Geometry: final body of the model. Coordinates: model frame, mm. Give positions to 0.01 mm unless a question says otherwise; leave off trailing zeros. Order: outer loops, then holes, each group sorted by start corner. A loop starts at its lowest first (then second) coordinate and runs counter-clockwise, first axis right, second up. Notation, with made-up numbers: (16.25, 20) -> (43.25, 20) arc R21 cw to (43.25, 53) -> close; hole circle Ø2 at (83.25, 57). An arc over 180 degrees is marked (long way). One line per question, with ' | ' between items.
from build123d import *

# Parameters (mm, degrees)
SKETCH1_W           = 1.5875
SKETCH1_H           = 1.7272
SKETCH1_R           = 1.0541
SKETCH1_H_2         = 1.778
BOSS_EXTRUDE1_DEPTH = 1.5875


with BuildPart() as part:
    # Sketch1 → Boss-Extrude1 (new body)
    with BuildSketch(Plane.XY):
        with BuildLine():
            Line((-20.6375, 22.848075056), (-20.6375, 0))
            Line((-20.6375, 0), (20.6375, 0))
            Line((20.6375, 0), (20.6375, 38.1))
            Line((20.6375, 38.1), (-20.6375, 38.1))
            Line((-20.6375, 38.1), (-20.6375, 33.337040193))
            ThreePointArc((-20.6375, 33.337040193), (-18.972227818, 30.628064614), (-19.079863508, 27.45))
            Line((-19.079863508, 27.45), (-20.6375, 22.848075056))
        make_face()
        with Locations((-17.68475, 2.977543878)):
            Rectangle(SKETCH1_W, SKETCH1_H, mode=Mode.SUBTRACT)
        with Locations((-18.4658, 14.5415)):
            Circle(SKETCH1_R, mode=Mode.SUBTRACT)
        with Locations((-17.68475, 18.002943878)):
            Rectangle(SKETCH1_W, SKETCH1_H_2, mode=Mode.SUBTRACT)
        with Locations((14.50975, 2.977543878)):
            Rectangle(SKETCH1_W, SKETCH1_H, mode=Mode.SUBTRACT)
        with Locations((14.50975, 18.002943878)):
            Rectangle(SKETCH1_W, SKETCH1_H_2, mode=Mode.SUBTRACT)
        with Locations((18.4658, 14.5415)):
            Circle(SKETCH1_R, mode=Mode.SUBTRACT)
        with BuildLine():
            Line((-8.4, 17), (-8.4, 23.35))
            Line((-8.4, 23.35), (-10.7, 23.35))
            ThreePointArc((-10.7, 23.35), (-12.75, 25.4), (-10.7, 27.45))
            Line((-10.7, 27.45), (-8.4, 27.45))
            Line((-8.4, 27.45), (-8.4, 33.8))
            Line((-8.4, 33.8), (8.4, 33.8))
            Line((8.4, 33.8), (8.4, 27.45))
            Line((8.4, 27.45), (10.7, 27.45))
            ThreePointArc((10.7, 27.45), (12.75, 25.4), (10.7, 23.35))
            Line((10.7, 23.35), (8.4, 23.35))
            Line((8.4, 23.35), (8.4, 17))
            Line((8.4, 17), (-8.4, 17))
        make_face(mode=Mode.SUBTRACT)
        with Locations((-18.4658, 36.2585)):
            Circle(SKETCH1_R, mode=Mode.SUBTRACT)
        with Locations((18.4658, 36.2585)):
            Circle(SKETCH1_R, mode=Mode.SUBTRACT)
    extrude(amount=BOSS_EXTRUDE1_DEPTH)


solid = part.part
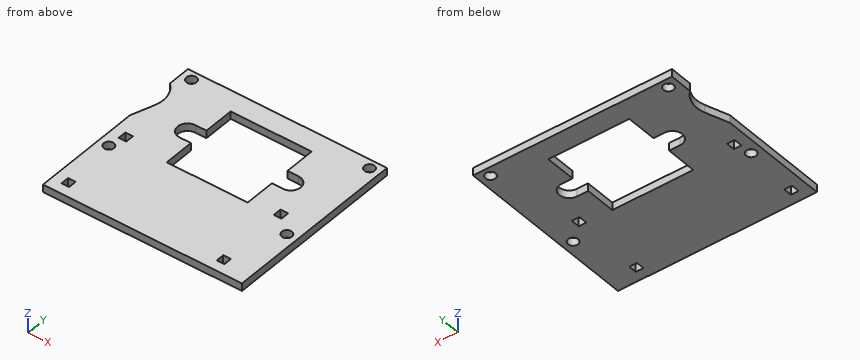
1) Section B-B on x = 5.5. Return loops of the section in (y, z).
Check result:
outline: (0, 0) -> (17, 0) -> (17, 1.59) -> (0, 1.59) -> close; (33.8, 0) -> (38.1, 0) -> (38.1, 1.59) -> (33.8, 1.59) -> close
2) Section A-A on y = 20. Return loops of the section in (x, z), plus the area to 3 significant figures.
Check result:
outline: (-20.64, 0) -> (-8.4, 0) -> (-8.4, 1.59) -> (-20.64, 1.59) -> close; (8.4, 0) -> (20.64, 0) -> (20.64, 1.59) -> (8.4, 1.59) -> close | area: 38.9 mm^2
3) Section C-C on z = 0.8. Count the separate pieces of the cut face and the enclosed holes in it, plus the area to 3 significant figures.
Check result:
separate pieces: 1 | enclosed holes: 9 | area: 1,220 mm^2
4) Material intervals for probe 1 along Y at (x, z) = (14, 1.5); probe 2 along Y at (x, z) = (5.5, 0.7); probe 3 along X at (y, z) = (31, 1.3), sorted ascending. Write a range as from..to.
Check result:
probe 1: y = 0..2.11, 3.84..17.11, 18.89..38.1 | probe 2: y = 0..17, 33.8..38.1 | probe 3: x = -19.08..-8.4, 8.4..20.64
